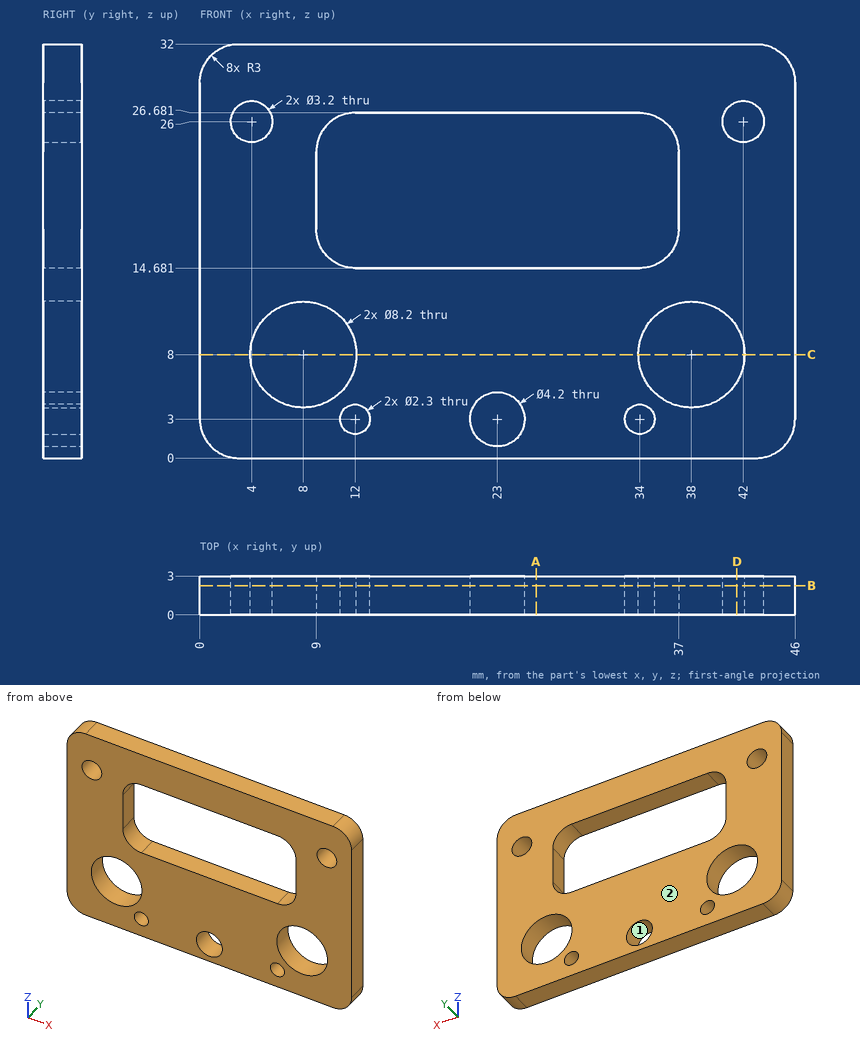
Geometry check sheet. Reference: drawing and pictorial views, mm from the part's lowest x, y, z. Give positions to 0.01 mm unless a question says otherwise; leave off trailing zeros. Loops run counter-clockwise (first coordinate to the right, second up) from the corner with the lowest first, then second, coordinate; pieces in that order, holes last. Notation, with made-up numbers: M 56,-13.75 L 79,-13.75 A23 cw 79,2.25 Z; hole C 71.25,20 d5. An arc over 180 degrees is marked long. Use a Markdown table: item, result. Add a question column.
Q1. Sectioned sample at D-D, the plane x = 41.5. Record the cut outline in (y, z).
Q2. Sectioned sample at B-B, the plane y = 2.25. Give the number of separate pieces and of enclosed holes in the cut face, then the cut area to 3 significant figures.
Q3. Sectioned sample at C-C, the plane z = 8. Record the cut outline in (x, y), then the cut area to 3 significant figures.
Q4. Sectioned sample at A-A, the plane x = 26. Record the cut outline in (y, z), then the cut area to 3 significant figures.
Q5. Scan lines: line 1 along X through (y, z) = (2, 8); line 2 along X through (y, z) = (1.8, 3); line 3 along Z through (x, y) = (13, 0.7). Record each from-to range of solid material in increasing order. Write a range as [from, to].
Q6. Mould release check, pull along X, two halves, no side actions. Record for the marked faces 1 and 2: pulls with the +X half, pulls with the -X half, needs draft (parallel to the pull), parting line crosses it, or undercut.
Q7. Go/stop test with flat-tipped pins: pin 1 (9.5 mm diameter, centred on x = 38, z = 8, fed in from +Y); pin 2 (1.9 mm diameter, centred on x = 42, z = 26, fed in from +Y). Record where each tip stops, or that it passes through.
Verdict:
| question | item | result |
|---|---|---|
| 1 | outline | M 0,0 L 3,0 L 3,5.86 L 0,5.86 Z; M 0,10.14 L 3,10.14 L 3,24.48 L 0,24.48 Z; M 0,27.52 L 3,27.52 L 3,32 L 0,32 Z |
| 2 | separate pieces | 1 |
| 2 | enclosed holes | 8 |
| 2 | area | 992 mm^2 |
| 3 | outline | M 0,0 L 3.9,0 L 3.9,3 L 0,3 Z; M 12.1,0 L 33.9,0 L 33.9,3 L 12.1,3 Z; M 42.1,0 L 46,0 L 46,3 L 42.1,3 Z |
| 3 | area | 88.8 mm^2 |
| 4 | outline | M 0,0 L 3,0 L 3,14.68 L 0,14.68 Z; M 0,26.68 L 3,26.68 L 3,32 L 0,32 Z |
| 4 | area | 60.0 mm^2 |
| 5 | line 1 | [0, 3.9], [12.1, 33.9], [42.1, 46] |
| 5 | line 2 | [0, 10.85], [13.15, 20.9], [25.1, 32.85], [35.15, 46] |
| 5 | line 3 | [0, 2.43], [3.57, 14.68], [26.68, 32] |
| 6 | face 1 | undercut |
| 6 | face 2 | needs draft |
| 7 | pin 1 | y = 3 |
| 7 | pin 2 | through |
